```python
from build123d import *

# Parameters (mm, degrees)
F1_DEPTH = 12.7
F1_TAPER = 12.5


with BuildPart() as f1:
    # F0 (on Front) → F1 (new body)
    with BuildSketch(Plane.XZ):
        with BuildLine():
            Line((50.8, -44.45), (35.9927948345, -44.45))
            ThreePointArc((35.9927948345, -44.45), (35.9688528047, -44.4330816985), (35.9768051433, -44.4048645047))
            ThreePointArc((35.9768051433, -44.4048645047), (0, 57.15), (-35.9768051433, -44.4048645047))
            ThreePointArc((-35.9768051433, -44.4048645047), (-35.9688528047, -44.4330816985), (-35.9927948345, -44.45))
            Line((-35.9927948345, -44.45), (-50.8, -44.45))
            Line((-50.8, -44.45), (-50.8, -69.85))
            Line((-50.8, -69.85), (50.8, -69.85))
            Line((50.8, -69.85), (50.8, -44.45))
        make_face()
        with BuildLine():
            ThreePointArc((-31.9297995416, -39.5111111111), (0, 50.8), (31.9297995416, -39.5111111111))
            ThreePointArc((31.9297995416, -39.5111111111), (29.9341870702, -46.5666666667), (35.9210244843, -50.8))
            Line((35.9210244843, -50.8), (44.45, -50.8))
            Line((44.45, -50.8), (44.45, -63.5))
            Line((44.45, -63.5), (-44.45, -63.5))
            Line((-44.45, -63.5), (-44.45, -50.8))
            Line((-44.45, -50.8), (-35.9210244843, -50.8))
            ThreePointArc((-35.9210244843, -50.8), (-29.9341870702, -46.5666666667), (-31.9297995416, -39.5111111111))
        make_face(mode=Mode.SUBTRACT)
    extrude(amount=F1_DEPTH, taper=F1_TAPER)


solid = f1.part
```
Read the model definition and answer for the solid it produces. Units are mm, in the model's axes. Coordinates: 2 decimals unless noted, no trailing zeros. Write each loop counter-clockwise with the first axis right and the second up, starting at its lowest first coordinate (ties: lowest second). Pieces come first, ordered by that corner, then holes. Notation, with made-up numbers: (-1, 10.5) -> (31, 10.5) arc R20 cw to (31, 20.5) -> close; hole circle Ø11 at (-9, -24.75). An arc over 180 degrees is marked (long way). Write item = value, one per line.
(1) Given pin 1 Ø1.5 at (x, y) = (30.5, -3.5) entering from +Z; pin 2 Ø2 at (y, z) = (-8.5, -55.5) entering from +X; pin 3 Ø5 at (x, y) = (-26, -1.5) entering from +Z, each flat-ended and moving along its own axis, determine where each tip first touches the part or whether it passes through.
From the geometry:
pin_1 = 47.92
pin_2 = 49.14
pin_3 = 51.88
(2) Straight lines are drawn through the part: L1, parallel to Z at x = 48, y = -5; L2, parallel to Z at x = -48, y = -8.5; L3, parallel to X at y = -8, z = -52.5. For each, find the intervals that lie inside material, in ascending order. Write a range as from..to.
From the geometry:
L1 = -68.74..-45.56, -28.92..-19.76, 19.76..28.92
L2 = -67.97..-46.33, -27.39..-21.72, 21.72..27.39
L3 = -49.03..-46.22, 46.22..49.03
(3) Section A-A on z = 0 is taken. Write down the section's boundary in (x, y), plus the area to 3 significant figures.
From the geometry:
outline = (-57.15, 0) -> (-54.33, -12.7) -> (-53.62, -12.7) -> (-50.8, 0) -> close; (50.8, 0) -> (53.62, -12.7) -> (54.33, -12.7) -> (57.15, 0) -> close
area = 89.8 mm2
